```python
from build123d import *

# Parameters (mm, degrees)
F0_W     = 182.557866
F0_H     = 170.73226
F2_DEPTH = 152.4
F3_R     = 32.274979
F4_DEPTH = 187.378392


with BuildPart() as f2:
    # F0 (on Top) → F2 (new body)
    with BuildSketch(Plane.XY):
        with Locations((-43.606944, 41.759193)):
            Rectangle(F0_W, F0_H)
    extrude(amount=F2_DEPTH)

    # F3
    f3_edges = [f2.edges().sort_by_distance(p)[0] for p in [
        (-43.606944, 127.125323, 152.4),
        (47.671989, 41.759193, 152.4),
        (-43.606944, -43.606937, 152.4),
        (-134.885877, 41.759193, 152.4),
    ]]
    fillet(f3_edges, radius=F3_R)

    # F1 (on face) → F4 (cut)
    with BuildSketch(Plane.XY):
        Polygon((-134.885877, -43.606937), (-134.885877, 80.69703), (-209.891543, 80.69703), (-209.891543, -80.69703), (0, -80.69703), (0, -43.606937), align=None)
    extrude(amount=F4_DEPTH, mode=Mode.SUBTRACT)


solid = f2.part
```
Geometry: final body of the model. Coordinates: model frame, mm. Round coordinates to 2 decimals unless told otherwise and drop trailing zeros. Loops run counter-clockwise (first coordinate to the right, second up) from the corner with the lowest first, then second, coordinate; pieces in that order, holes last. Notation, with made-up numbers: (-15.75, 11) -> (-7.75, 11) arc R5 ccw to (-7.75, 17) -> close; hole circle Ø8 at (61, 5.5). An arc over 180 degrees is marked (long way). Use one line per item in the form item = value. Start each with the question number.
1) Section C-C on z = 132. Output: boundary loops of the cut face in (x, y).
2) Section B-B on y = 86. Output: boundary loops of the cut face in (x, z), then the cut area to 3 significant figures.
3) First-contact query: P1, Ø8, axis at x = 27.5, z = 126, coming from the -Y side; P2, Ø2, axis at x = -26, y = 99.5, coming from the +Z side; P3, Ø3, axis at x = -33, y = 99, coming from the +Z side. Flat tips, straight axial feed; report the tip coordinate or a pass-through.
4) Line query: L1, parallel to Z at x = -103.5, y = 34.5; L2, parallel to X at y = 28, z = 138; L3, parallel to Y at x = 5, z = 123. Output: solid intervals per line, ascending.
5) Section A-A on x = -37. Output: boundary loops of the cut face in (y, z), then the cut area to 3 significant figures.
Response:
q1.outline = (-132.62, -41.34) -> (45.41, -41.34) -> (45.41, 124.86) -> (-132.62, 124.86) -> close
q2.outline = (-134.89, 0) -> (47.67, 0) -> (47.67, 120.13) arc R32.27 ccw to (15.4, 152.4) -> (-102.61, 152.4) arc R32.27 ccw to (-134.89, 120.13) -> close
q2.area = 27,400 mm^2
q3.P1 = -43.55
q3.P2 = 152.19
q3.P3 = 152.29
q4.L1 = 0 to 152.39
q4.L2 = -129.48 to 42.27
q4.L3 = -43.48 to 127
q5.outline = (-43.61, 0) -> (127.13, 0) -> (127.13, 120.13) arc R32.27 ccw to (94.85, 152.4) -> (-11.33, 152.4) arc R32.27 ccw to (-43.61, 120.13) -> close
q5.area = 25,600 mm^2
